Can you work these out from the model? Positions are in its coordinate system, mm. A direction names the side the tool comes from. Coordinates: 2 decimals unless noted, no trailing zeros. Order: outer loops, then holes, each group sorted by start corner. A loop starts at its lowest first (then second) coordinate and runs counter-clockwise, first axis right, second up. Notation, with made-up numbers: (-5, 66) -> (2, 66) arc R17 ccw to (2, 81) -> close; hole circle Ø7 at (8.25, 86.5). An arc over 180 degrees is marked (long way). Answer as a JSON object with one key per item and string values. Group by question number.
(1) I need wall thicknesses on line 1 (Z direction, x = 0.2, y = -34); line 2 (Y direction, x = 1.8, z = 14); line 3 (Z direction, x = 4.8, y = -8). Which ranges of each line are inside material? Lowest first, please.
(2) I want a section at A-A, the plane y = 9. List the corners of the cut face in (x, z) for me, plus the area to 3 significant figures.
(3) I want a section at D-D, the plane y = -22.5. List the corners of the cut face in (x, z) for me, plus the area to 3 significant figures.
(4) If we mould it in two halves opening along Y, with no side actions, what happens to faces 6 (the cylindrical face through (2.535, -18.915, 28.841)), 7 (the flat face through (2, 0, -35)), 8 (the flat face through (2, 35, -23))? For each: pulls with the +Y half, pulls with the -Y half, needs draft (parallel to the pull), parting line crosses it, or undercut.
(5) Which directions (+Z, -Z, +X, -X, +Y, -Y) give clear straight access to the entire face, cutting with the end or side of a thin tool? Please do faces 1 (the flat face through (2, 20, -33)), 2 (the flat face through (2, -20, 33)), 3 (the flat face through (2, 35, 23)), 4 (the flat face through (3, -11, -5)), 5 (the flat face through (5, 1, 8)).
(6) I want a section at C-C, the plane z = -26. List the corners of the cut face in (x, y) for me.
(7) For pin 1 (1.5 mm diameter, centred on x = 3, z = 22, fed in from -Y); pin 2 (1.9 mm diameter, centred on y = 35, z = -15, fed in from +X); pin 3 (1.5 mm diameter, centred on x = 3.5, y = 28.5, fed in from -Z); pin 4 (1 mm diameter, centred on x = 3, z = -33, fed in from -Y), each with a flat end and sliding along its axis, tell me the tip position at first contact or that it passes through.
from build123d import *

# Parameters (mm, degrees)
SKETCH1_W                                = 70
SKETCH1_H                                = 80
BOSS_EXTRUDE1_DEPTH                      = 5
CUT_EXTRUDE1_START                       = -6
CUT_EXTRUDE1_DEPTH                       = 7
MIRROR1_START                            = -6
MIRROR1_AT_THE_SECOND_PLANE_COPY_1_DEPTH = 7
CUT_EXTRUDE2_DEPTH                       = 1
CUT_EXTRUDE2_DEPTH_BACK                  = 6
SKETCH5_R                                = 1.5875
CUT_EXTRUDE3_DEPTH                       = 6


with BuildPart() as part:
    # Sketch1 → Boss-Extrude1 (new body)
    with BuildSketch(Plane(origin=(0, 0, 0), x_dir=(0, 0, -1), z_dir=(1, 0, 0))):
        Rectangle(SKETCH1_W, SKETCH1_H)
    extrude(amount=BOSS_EXTRUDE1_DEPTH)

    # Sketch3 → Cut-Extrude1 (cut)
    with BuildSketch(Plane(origin=(5, 0, 0), x_dir=(0, 0, -1), z_dir=(1, 0, 0)).offset(CUT_EXTRUDE1_START)):
        Polygon((-35, 20), (-30, 20), (-30, 35), (-15, 35), (-15, 40), (-35, 40), align=None)
    cut_extrude1 = extrude(amount=CUT_EXTRUDE1_DEPTH, mode=Mode.SUBTRACT)

    # Mirror1: Cut-Extrude1 across plane
    add(cut_extrude1.mirror(Plane.XY), mode=Mode.SUBTRACT)

    # Mirror1 at the second plane: Cut-Extrude1 across plane
    add(cut_extrude1.mirror(Plane.ZX), mode=Mode.SUBTRACT)

    # Mirror1 at the second plane copy 1 sketc → Mirror1 at the second plane copy 1 (cut)
    with BuildSketch(Plane(origin=(5, 0, 0), x_dir=(0, 0, 1), z_dir=(1, 0, 0)).offset(MIRROR1_START)):
        Polygon((-35, 20), (-30, 20), (-30, 35), (-15, 35), (-15, 40), (-35, 40), align=None)
    extrude(amount=MIRROR1_AT_THE_SECOND_PLANE_COPY_1_DEPTH, mode=Mode.SUBTRACT)

    # Sketch4 → Cut-Extrude2 (cut, two sides)
    with BuildSketch(Plane(origin=(5, 0, 0), x_dir=(0, 0, -1), z_dir=(1, 0, 0))) as cut_extrude2_sk:
        with BuildLine():
            Line((-3, -40), (5, -40))
            Line((5, -40), (5, 18.4125))
            ThreePointArc((5, 18.4125), (4.535032015, 19.535032015), (3.4125, 20))
            Line((3.4125, 20), (-1.4125, 20))
            ThreePointArc((-1.4125, 20), (-2.535032015, 19.535032015), (-3, 18.4125))
            Line((-3, 18.4125), (-3, -40))
        make_face()
    extrude(amount=CUT_EXTRUDE2_DEPTH, mode=Mode.SUBTRACT)
    extrude(cut_extrude2_sk.sketch, amount=-CUT_EXTRUDE2_DEPTH_BACK, mode=Mode.SUBTRACT)

    # Sketch5 → Cut-Extrude3 (cut, through all)
    with BuildSketch(Plane(origin=(5, 0, 0), x_dir=(0, 0, -1), z_dir=(1, 0, 0))):
        with Locations((-15, 35)):
            Circle(SKETCH5_R)
        with Locations((15, 35)):
            Circle(SKETCH5_R)
        with Locations((30, 20)):
            Circle(SKETCH5_R)
        with Locations((30, -20)):
            Circle(SKETCH5_R)
        with Locations((15, -35)):
            Circle(SKETCH5_R)
        with Locations((-15, -35)):
            Circle(SKETCH5_R)
        with Locations((-30, -20)):
            Circle(SKETCH5_R)
        with Locations((-30, 20)):
            Circle(SKETCH5_R)
    extrude(amount=-CUT_EXTRUDE3_DEPTH, mode=Mode.SUBTRACT)


solid = part.part
Computed values:
{
 "1": {"line 1": "z = -30 to -16.23, -13.77 to -5, 3 to 13.77, 16.23 to 30", "line 2": "y = -40 to -36.23, -33.77 to 33.77, 36.23 to 40", "line 3": "z = -35 to -5, 3 to 35"},
 "2": {"outline": "(0, -35) -> (5, -35) -> (5, -5) -> (0, -5) -> close; (0, 3) -> (5, 3) -> (5, 35) -> (0, 35) -> close", "area": "310 mm2"},
 "3": {"outline": "(0, -30) -> (5, -30) -> (5, -5) -> (0, -5) -> close; (0, 3) -> (5, 3) -> (5, 30) -> (0, 30) -> close", "area": "260 mm2"},
 "4": {"face 6": "undercut", "face 7": "needs draft", "face 8": "pulls with the +Y half"},
 "5": {"face 1": "-Z, +X, -X, +Y", "face 2": "+Z, +X, -X, -Y", "face 3": "+Z, +X, -X, +Y", "face 4": "+X, -X, -Y", "face 5": "+Z, -Z, +X, +Y, -Y"},
 "6": {"outline": "(0, -35) -> (5, -35) -> (5, 35) -> (0, 35) -> close"},
 "7": {"pin 1": "stops at y = -35", "pin 2": "passes through", "pin 3": "stops at z = -30", "pin 4": "stops at y = -20"}
}
